Check sheet for the modelled part. Datum: model origin and axes. Units: mm. Face numbers are marked on the shaded views. Give positions to 0.01 mm unless a question says otherwise; leave off trailing zeros. Order: outer loops, then holes, each group sorted by start corner. A loop starts at its lowest first (then second) coordinate and runs counter-clockwise, first axis right, second up. Notation, with made-up numbers: (53.5, 77) - (108.5, 77) arc R9 ccw to (108.5, 88) - close; hole circle Ø5 at (49.5, 56). An arc over 180 degrees is marked (long way). Answer in a Markdown table with one row per item.
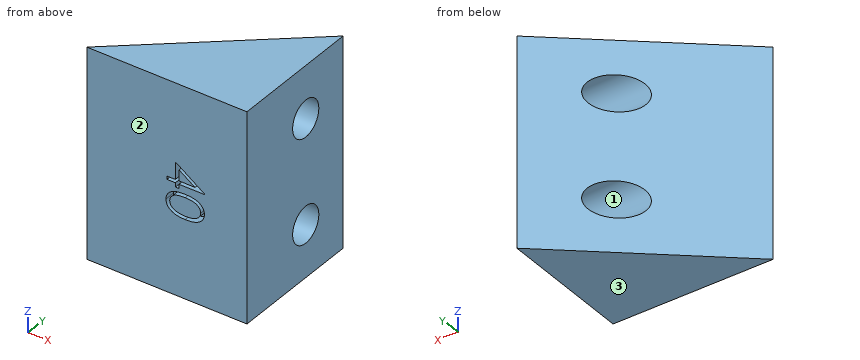
from build123d import *

# Parameters (mm, degrees)
BOSS_EXTRUDE1_DEPTH = 20
CUT_EXTRUDE1_REACH  = 30.284
SKETCH3_R           = 1.75
CUT_EXTRUDE2_DEPTH  = 1


with BuildPart() as part:
    # Sketch1 → Boss-Extrude1 (new body)
    with BuildSketch(Plane.XY):
        Polygon((0, 0), (-15.320888862, 0), (0, 12.855752194), align=None)
    extrude(amount=BOSS_EXTRUDE1_DEPTH)

    # Cut-Extrude1: up to this plane
    cut_extrude1_end = Plane(origin=(-15.320888862, 0, 20), z_dir=(0.6427876096865347, -0.7660444431189819, 0))
    # Sketch3 → Cut-Extrude1 (cut, up to the surface)
    with BuildSketch(Plane(origin=(0, 0, 0), x_dir=(0, 0, -1), z_dir=(1, 0, 0)), mode=Mode.PRIVATE) as cut_extrude1_sk1:
        with Locations(Location((-5, 7.855752194, 0), (0, 0, 90))):
            Circle(SKETCH3_R)
    cut_extrude1_tool1 = split(extrude(cut_extrude1_sk1.sketch, amount=-CUT_EXTRUDE1_REACH, mode=Mode.PRIVATE), bisect_by=cut_extrude1_end, keep=Keep.BOTH, mode=Mode.PRIVATE)
    add(cut_extrude1_tool1.solids().sort_by_distance((0, 7.855752, 5))[0], mode=Mode.SUBTRACT)
    # Sketch3 → Cut-Extrude1 (cut, up to the surface)
    with BuildSketch(Plane(origin=(0, 0, 0), x_dir=(0, 0, -1), z_dir=(1, 0, 0)), mode=Mode.PRIVATE) as cut_extrude1_sk2:
        with Locations(Location((-15, 7.855752194, 0), (0, 0, 90))):
            Circle(SKETCH3_R)
    cut_extrude1_tool2 = split(extrude(cut_extrude1_sk2.sketch, amount=-CUT_EXTRUDE1_REACH, mode=Mode.PRIVATE), bisect_by=cut_extrude1_end, keep=Keep.BOTH, mode=Mode.PRIVATE)
    add(cut_extrude1_tool2.solids().sort_by_distance((0, 7.855752, 15))[0], mode=Mode.SUBTRACT)

    # Sketch4 → Cut-Extrude2 (cut)
    # profile 1 of 2: a face of its own
    with BuildSketch(Plane.XZ):
        with BuildLine():
            add(Edge.make_bspline(
                [(-5.911846675, 9.865384615), (-5.855749287, 9.865056597), (-5.746779303, 9.864419417), (-5.587994661, 9.857330996), (-5.439034371, 9.845555655), (-5.299891307, 9.829418279), (-5.170529535, 9.809780308), (-5.051294804, 9.783564792), (-4.941635109, 9.753752086), (-4.841193358, 9.719199315), (-4.748614631, 9.680212646), (-4.662193041, 9.637774437), (-4.582038305, 9.590223642), (-4.506946286, 9.540196681), (-4.437755047, 9.485865435), (-4.374595619, 9.427802965), (-4.317429865, 9.365433315), (-4.265577415, 9.299990015), (-4.220407322, 9.231059481), (-4.179706065, 9.160766611), (-4.146300055, 9.087871031), (-4.118851035, 9.013037572), (-4.096856831, 8.936483858), (-4.081625887, 8.857893574), (-4.07208018, 8.777247733), (-4.071164983, 8.72281691), (-4.070700841, 8.69521234)],
                knots=[0, 0, 0, 0, 1.646377244, 3.198111528, 4.663803227, 6.031090796, 7.308794487, 8.502186765, 9.612154809, 10.642545331, 11.617106989, 12.558866172, 13.465886467, 14.35053239, 15.20542558, 16.045215227, 16.865619885, 17.686225247, 18.492864914, 19.282407821, 20.068097601, 20.842842034, 21.620163247, 22.403093475, 23.190129512, 24, 24, 24, 24], degree=3))
            add(Edge.make_bspline(
                [(-4.070700841, 8.69521234), (-4.071188657, 8.667376861), (-4.072158768, 8.612020852), (-4.08148271, 8.530180477), (-4.096953833, 8.450230795), (-4.118874808, 8.372512657), (-4.146070484, 8.29638767), (-4.180157602, 8.222451263), (-4.219836469, 8.150244181), (-4.266460346, 8.080913893), (-4.318442622, 8.013699278), (-4.377205291, 7.950251315), (-4.44215501, 7.890564229), (-4.512596874, 7.833888924), (-4.589881959, 7.781833327), (-4.672666069, 7.732259894), (-4.762396934, 7.687887858), (-4.857577402, 7.645153183), (-4.96084106, 7.608266197), (-5.071605821, 7.574999951), (-5.191180008, 7.548120983), (-5.318936253, 7.52573171), (-5.455343736, 7.508386814), (-5.600110052, 7.495754172), (-5.753330442, 7.489081087), (-5.858088292, 7.487824386), (-5.911846675, 7.487179487)],
                knots=[0, 0, 0, 0, 0.810914788, 1.612654377, 2.396697861, 3.181598691, 3.963628158, 4.749916497, 5.551656086, 6.361998678, 7.18212741, 8.025565596, 8.878627764, 9.750805457, 10.657531673, 11.591944965, 12.560506719, 13.57287815, 14.630710178, 15.753379473, 16.941251878, 18.199788006, 19.531962791, 20.947069417, 22.433333509, 24, 24, 24, 24], degree=3))
            add(Edge.make_bspline(
                [(-5.911846675, 7.487179487), (-5.965370383, 7.487831877), (-6.069659145, 7.489103032), (-6.222192885, 7.495670613), (-6.366181214, 7.508668333), (-6.502024942, 7.524744462), (-6.628917519, 7.547644686), (-6.748065541, 7.573678205), (-6.85844078, 7.606035075), (-6.961159835, 7.64241929), (-7.05587398, 7.684226665), (-7.144829164, 7.728990868), (-7.227545725, 7.778260008), (-7.304829686, 7.830626053), (-7.375882464, 7.886819625), (-7.440879663, 7.946759451), (-7.499778411, 8.010491153), (-7.552470928, 8.077857734), (-7.598552071, 8.148278684), (-7.6397412, 8.220244748), (-7.673163625, 8.295192302), (-7.701382826, 8.371455698), (-7.723354231, 8.449754531), (-7.738397903, 8.530012), (-7.748977846, 8.611965265), (-7.749783232, 8.667367231), (-7.750188021, 8.69521234)],
                knots=[0, 0, 0, 0, 1.56130642, 3.042141888, 4.451772327, 5.777565838, 7.030558081, 8.211376819, 9.333164717, 10.383253789, 11.387583522, 12.350962576, 13.286244149, 14.193812918, 15.072134482, 15.925989337, 16.770211267, 17.600669898, 18.417446232, 19.22325363, 20.01647746, 20.807971184, 21.593601364, 22.38506573, 23.188331689, 24, 24, 24, 24], degree=3))
            add(Edge.make_bspline(
                [(-7.750188021, 8.69521234), (-7.749719413, 8.722815788), (-7.748795409, 8.777244401), (-7.739314215, 8.857906439), (-7.723853582, 8.936374154), (-7.702858119, 9.012804408), (-7.67617413, 9.087353616), (-7.642233085, 9.159291496), (-7.602866753, 9.2295681), (-7.558080183, 9.297862753), (-7.50675594, 9.3628738), (-7.449992852, 9.424973717), (-7.386367185, 9.482594504), (-7.316897365, 9.536244807), (-7.242172844, 9.58715603), (-7.161457528, 9.634240862), (-7.074226219, 9.676596293), (-6.981136428, 9.716456686), (-6.87995648, 9.751593547), (-6.769711906, 9.782396514), (-6.649792857, 9.808075096), (-6.520555338, 9.828725945), (-6.38190262, 9.845750492), (-6.233590578, 9.857275238), (-6.075747171, 9.864425062), (-5.967477141, 9.865058928), (-5.911846675, 9.865384615)],
                knots=[0, 0, 0, 0, 0.810940842, 1.599017053, 2.38298203, 3.159479784, 3.926441347, 4.70693857, 5.494146311, 6.292334103, 7.104379492, 7.925868426, 8.762126819, 9.623561095, 10.503686106, 11.41783325, 12.366995289, 13.351843594, 14.392337808, 15.512229747, 16.713911458, 17.994391108, 19.357476964, 20.818259213, 22.365182633, 24, 24, 24, 24], degree=3))
        make_face()
        with BuildLine():
            add(Edge.make_bspline(
                [(-5.910444431, 9.551282051), (-5.95719313, 9.551162604), (-6.047923175, 9.550930781), (-6.179766436, 9.54487458), (-6.302736765, 9.536624349), (-6.416990299, 9.525983049), (-6.52214032, 9.51018011), (-6.618909975, 9.492473291), (-6.706787304, 9.470925304), (-6.786374812, 9.445429949), (-6.859024912, 9.416392001), (-6.926622524, 9.384682123), (-6.989987212, 9.350635607), (-7.048475401, 9.312465852), (-7.102669298, 9.271038631), (-7.152413166, 9.226285917), (-7.19748996, 9.178286418), (-7.250977945, 9.111839375), (-7.306904454, 9.024548906), (-7.355005521, 8.914002071), (-7.3854296, 8.800360685), (-7.389287877, 8.723205872), (-7.391213662, 8.684695513)],
                knots=[0, 0, 0, 0, 1.459116078, 2.831857795, 4.118796693, 5.306371758, 6.412361096, 7.436813035, 8.376339383, 9.234574298, 10.043323891, 10.816788787, 11.564361537, 12.286735248, 12.994408768, 13.691741332, 14.372975427, 15.047457468, 16.352811911, 17.594285292, 18.799233213, 20, 20, 20, 20], degree=3))
            add(Edge.make_bspline(
                [(-7.391213662, 8.684695513), (-7.389615881, 8.645937841), (-7.386423618, 8.568502518), (-7.355624881, 8.455368723), (-7.309155342, 8.345538453), (-7.254207836, 8.259466512), (-7.201879507, 8.193983969), (-7.157264858, 8.147066979), (-7.107308991, 8.10400493), (-7.053409695, 8.063162856), (-6.994537211, 8.02570378), (-6.930974636, 7.991640642), (-6.862545458, 7.960557295), (-6.814775719, 7.942848249), (-6.790352284, 7.933794071)],
                knots=[0, 0, 0, 0, 1.353760809, 2.704726607, 4.075137775, 5.516104923, 6.260822281, 7.007110065, 7.778089737, 8.566572457, 9.372053459, 10.217411131, 11.088608312, 12, 12, 12, 12], degree=3))
            add(Edge.make_bspline(
                [(-6.790352284, 7.933794071), (-6.759122544, 7.923242303), (-6.69571278, 7.901817689), (-6.597349128, 7.874205915), (-6.494146364, 7.852460515), (-6.386721247, 7.83289715), (-6.274281546, 7.819544094), (-6.157175162, 7.80879628), (-6.0353138, 7.802465594), (-5.952518809, 7.801680842), (-5.910444431, 7.801282051)],
                knots=[0, 0, 0, 0, 0.884706709, 1.796334032, 2.740027952, 3.714592787, 4.726048262, 5.777819803, 6.87074269, 8, 8, 8, 8], degree=3))
            add(Edge.make_bspline(
                [(-5.910444431, 7.801282051), (-5.868370958, 7.801721875), (-5.786056068, 7.802582372), (-5.665629311, 7.80823591), (-5.551049969, 7.817320676), (-5.4422141, 7.829616707), (-5.339315419, 7.846496558), (-5.242206679, 7.866767579), (-5.150914061, 7.890533025), (-5.065202128, 7.9177927), (-4.985378952, 7.948513976), (-4.911270741, 7.982451775), (-4.842484619, 8.018668005), (-4.779218028, 8.058011632), (-4.721185397, 8.100006966), (-4.669550825, 8.145764604), (-4.622713851, 8.193468954), (-4.569251284, 8.260286147), (-4.514739588, 8.347760433), (-4.464573828, 8.456606082), (-4.435765535, 8.569876726), (-4.431703848, 8.64645018), (-4.4296752, 8.684695513)],
                knots=[0, 0, 0, 0, 1.313668642, 2.570134578, 3.763346207, 4.902004944, 5.98888779, 7.017888835, 7.998425394, 8.933058446, 9.82474457, 10.667209444, 11.476765193, 12.250262638, 12.991704352, 13.7104269, 14.401925311, 15.076585796, 16.378385137, 17.609787933, 18.806186071, 20, 20, 20, 20], degree=3))
            add(Edge.make_bspline(
                [(-4.4296752, 8.684695513), (-4.43170403, 8.72340773), (-4.435765385, 8.80090269), (-4.464498285, 8.915326021), (-4.514272533, 9.024947029), (-4.569603302, 9.111719517), (-4.621767413, 9.178452408), (-4.667129522, 9.225575145), (-4.717023873, 9.269629998), (-4.770988327, 9.311091733), (-4.829506015, 9.349224743), (-4.892861488, 9.383285193), (-4.960465382, 9.414976868), (-5.033098953, 9.444077159), (-5.112806444, 9.469336238), (-5.200240265, 9.491913196), (-5.297100307, 9.509609273), (-5.402544299, 9.525051618), (-5.516938287, 9.536825531), (-5.640192121, 9.544853401), (-5.77226338, 9.550941739), (-5.863461555, 9.551166342), (-5.910444431, 9.551282051)],
                knots=[0, 0, 0, 0, 1.207964612, 2.418129846, 3.655795183, 4.951004962, 5.620895151, 6.296795572, 6.989224116, 7.696855977, 8.419187164, 9.166715907, 9.940135271, 10.748837255, 11.607021648, 12.548275234, 13.5654991, 14.678641405, 15.874140913, 17.15372626, 18.533675393, 20, 20, 20, 20], degree=3))
        make_face(mode=Mode.SUBTRACT)
    # profile 2 of 2: a face of its own
    with BuildSketch(Plane.XZ):
        Polygon((-4.070700841, 10.647135417), (-4.070700841, 10.583333333), (-6.493777765, 10.583333333), (-6.493777765, 10.179487179), (-6.852752123, 10.179487179), (-6.852752123, 10.583333333), (-7.660444431, 10.583333333), (-7.660444431, 10.897435897), (-6.852752123, 10.897435897), (-6.852752123, 12.557692308), align=None)
        Polygon((-6.493777765, 10.897435897), (-4.973745713, 10.897435897), (-6.493777765, 11.940705128), align=None, mode=Mode.SUBTRACT)
    extrude(amount=-CUT_EXTRUDE2_DEPTH, mode=Mode.SUBTRACT)


solid = part.part
(1) Cross-section at C-C, the plane x = -2. Record the cut outline in (y, z).
Geometry says:
| item | result |
|---|---|
| outline | (0, 0) - (11.18, 0) - (11.18, 20) - (0, 20) - close; hole circle Ø3.5 at (7.86, 5); hole circle Ø3.5 at (7.86, 15) |
(2) Cross-section at B-B, the plane z = 5. Record the cut outline in (x, y), then the cut area to 3 significant figures.
Geometry says:
| item | result |
|---|---|
| outline | (-15.32, 0) - (0, 0) - (0, 6.11) - (-8.04, 6.11) - close; (-3.87, 9.61) - (0, 9.61) - (0, 12.86) - close |
| area | 77.6 mm² |
(3) Cross-section at A-A, the plane y = 7.25. Record the cut outline in (x, z), then the cut area to 3 significant figures.
Geometry says:
| item | result |
|---|---|
| outline | (-6.68, 0) - (0, 0) - (0, 3.36) - (-6.68, 3.36) - close; (-6.68, 6.64) - (0, 6.64) - (0, 13.36) - (-6.68, 13.36) - close; (-6.68, 16.64) - (0, 16.64) - (0, 20) - (-6.68, 20) - close |
| area | 89.7 mm² |
(4) Cross-section at D-D, the plane y = 11.75. Record the cut outline in (x, z), then the cut area to 3 significant figures.
Geometry says:
| item | result |
|---|---|
| outline | (-1.32, 0) - (0, 0) - (0, 20) - (-1.32, 20) - close |
| area | 26.4 mm² |
(5) Gauge pin test, flat ends, axial feed: P1, Ø3, axis at y = 7.86, z = 15, coming from the +X side; P2, Ø4, axis at x = -10.5, z = 5.5, coming from the +Y side. Record the tip position at first contact, or that the pin passes through.
Geometry says:
| item | result |
|---|---|
| P1 | through |
| P2 | y = 5.72 |
(6) Mould release check, pull along Z, two halves, no side actions. Record for the marked faces 1, 2 and 3: pulls with the +Z half, pulls with the -Z half, needs draft (parallel to the pull), parting line crosses it, or undercut.
Geometry says:
| item | result |
|---|---|
| face 1 | undercut |
| face 2 | needs draft |
| face 3 | pulls with the -Z half |
(7) Thickness scan on L1, parallel to Z at x = -2.25, y = 8.25; L2, parallel to Z at x = -1.25, y = 9; L3, parallel to Y at x = -5.25, z = 5. Record the ranges inside material, lowest first.
Geometry says:
| item | result |
|---|---|
| L1 | 0 to 3.29, 6.71 to 13.29, 16.71 to 20 |
| L2 | 0 to 3.68, 6.32 to 13.68, 16.32 to 20 |
| L3 | 0 to 6.11 |
